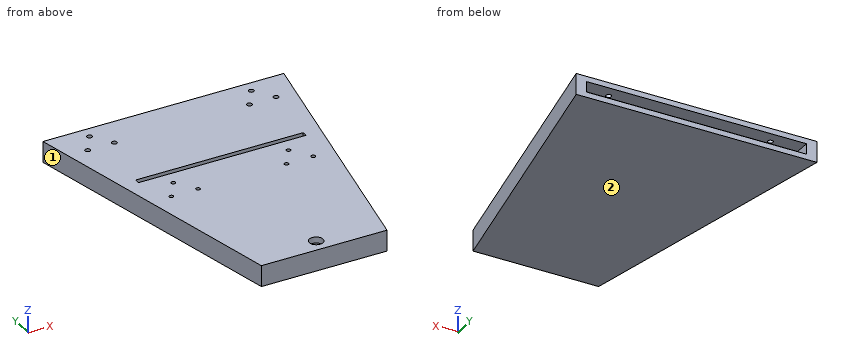
```python
from build123d import *

# Parameters (mm, degrees)
EXTRUDE_1_DEPTH     = 20
SKETCH_3_W          = 210
SKETCH_3_H          = 10
CUT_EXTRUDE_1_DEPTH = 15
SKETCH_4_W          = 160
SKETCH_4_H          = 5
CUT_EXTRUDE_2_DEPTH = 10
SKETCH_5_R          = 2.5
SKETCH_5_R_2        = 2
CUT_EXTRUDE_3_DEPTH = 10
CUT_EXTRUDE_4_DEPTH = 4.25
SKETCH_8_R          = 6.5
CUT_EXTRUDE_6_DEPTH = 15


with BuildPart() as part:
    # 草图1 → 凸台-拉伸1 (new body)
    with BuildSketch(Plane.XY):
        Polygon((-115, 220), (115, 220), (60, -50), (-60, -50), align=None)
    extrude(amount=EXTRUDE_1_DEPTH)

    # 草图3 → 切除-拉伸1 (cut)
    with BuildSketch(Plane(origin=(0, 220, 0), x_dir=(1, 0, 0), z_dir=(0, 1, 0))):
        with Locations((0, -10)):
            Rectangle(SKETCH_3_W, SKETCH_3_H)
    extrude(amount=-CUT_EXTRUDE_1_DEPTH, mode=Mode.SUBTRACT)

    # 草图4 → 切除-拉伸2 (cut)
    with BuildSketch(Plane.XY.offset(20)):
        with Locations((0, 123.51)):
            Rectangle(SKETCH_4_W, SKETCH_4_H)
    extrude(amount=-CUT_EXTRUDE_2_DEPTH, mode=Mode.SUBTRACT)

    # 草图5 → 切除-拉伸3 (cut)
    with BuildSketch(Plane.XY.offset(20)):
        with Locations((-77.25, 208.1425573)):
            Circle(SKETCH_5_R)
        with Locations((-90, 189)):
            Circle(SKETCH_5_R)
        with Locations((-64.5, 189)):
            Circle(SKETCH_5_R)
        with Locations((-55, 106.6525573)):
            Circle(SKETCH_5_R_2)
        with Locations((-67.75, 87.51)):
            Circle(SKETCH_5_R_2)
        with Locations((-42.25, 87.51)):
            Circle(SKETCH_5_R_2)
        with Locations(Location((42.25, 87.51, 0), (0, 0, 180))):
            Circle(SKETCH_5_R_2)
        with Locations(Location((67.75, 87.51, 0), (0, 0, 180))):
            Circle(SKETCH_5_R_2)
        with Locations(Location((55, 106.6525573, 0), (0, 0, 180))):
            Circle(SKETCH_5_R_2)
        with Locations(Location((64.5, 189, 0), (0, 0, 180))):
            Circle(SKETCH_5_R)
        with Locations(Location((90, 189, 0), (0, 0, 180))):
            Circle(SKETCH_5_R)
        with Locations((77.25, 208.1425573)):
            Circle(SKETCH_5_R)
    extrude(amount=-CUT_EXTRUDE_3_DEPTH, mode=Mode.SUBTRACT)

    # 草图6 → 切除-拉伸4 (cut, symmetric)
    with BuildSketch(Plane(origin=(0, 0, 10), x_dir=(-1, 0, 0), z_dir=(0, 0, -1))):
        with BuildLine():
            Line((0, -49.69), (18.016092171, -49.69))
            Line((18.016092171, -49.69), (11.781592332, -23.29))
            Line((11.781592332, -23.29), (0, -23.29))
            ThreePointArc((0, -23.29), (-13.2, -36.49), (0, -49.69))
        make_face()
    extrude(amount=CUT_EXTRUDE_4_DEPTH, both=True, mode=Mode.SUBTRACT)

    # 草图8 → 切除-拉伸6 (cut)
    with BuildSketch(Plane.XY.offset(20)):
        with Locations((0, -36.49)):
            Circle(SKETCH_8_R)
    extrude(amount=-CUT_EXTRUDE_6_DEPTH, mode=Mode.SUBTRACT)


solid = part.part
```
Build history of the part. All positions in model axes, mm. Face numbers are marked on the shaded views. Give positions to 0.01 mm unless a question says otherwise; leave off trailing zeros. Order: outer loops, then holes, each group sorted by start corner. A loop starts at its lowest first (then second) coordinate and runs counter-clockwise, first axis right, second up. Notation, with made-up numbers: M 11,65.5 L 49,65.5 A30 ccw 49,91.5 Z; hole C 13,46.5 d7. An arc over 180 degrees is marked long. Return JSON: item names as keys, results as strings.
Q1. Band-saw the part on D-D (y = 73). Give the cut face in (x, z).
Answer list:
{"outline": "M -85.06,0 L 85.06,0 L 85.06,20 L -85.06,20 Z"}
Q2. Wall check: probe 1 along Y at (x, z) = (-55, 15.5); probe 2 along X at (y, z) = (189, 17); probe 3 along Y at (x, z) = (-32.5, 9.75). Give the ranges that are in metal, low to high. Write a range as from..to.
Answer list:
{"probe 1": "y = -50..104.65, 108.65..121.01, 126.01..220", "probe 2": "x = -108.69..-92.5, -87.5..-67, -62..62, 67..87.5, 92.5..108.69", "probe 3": "y = -50..205"}
Q3. Two-plate mould, pull along X, no slides. Class the marked faces 1 and 2: pulls with the +X half, pulls with the -X half, needs draft (parallel to the pull), parting line crosses it, or undercut.
Answer list:
{"face 1": "pulls with the -X half", "face 2": "needs draft"}
Q4. Band-saw the part on A-A (x = -26). Give the cut face in (y, z).
Answer list:
{"outline": "M -50,0 L 220,0 L 220,5 L 205,5 L 205,15 L 220,15 L 220,20 L 126.01,20 L 126.01,10 L 121.01,10 L 121.01,20 L -50,20 Z"}
Q5. Flat gauge pins, fed straight in: pin 1 (1.5 mm diameter, centred on y = 122.5, z = 15, fed in from -X); pin 2 (3 mm diameter, centred on x = 36.5, z = 8.5, fed in from +Y); pin 3 (4 mm diameter, centred on y = 163.5, z = 8, fed in from +X). Where does each tip first touch, or does it go through?
Answer list:
{"pin 1": "stops at x = -95.29", "pin 2": "stops at y = 205", "pin 3": "stops at x = 103.9"}
Q6. Band-saw the part on B-B (y = -36.49). Give the cut face in (x, z).
Answer list:
{"outline": "M -62.75,0 L 62.75,0 L 62.75,20 L 6.5,20 L 6.5,14.25 L 13.2,14.25 L 13.2,5.75 L 6.5,5.75 L 6.5,5 L -6.5,5 L -6.5,5.75 L -14.9,5.75 L -14.9,14.25 L -6.5,14.25 L -6.5,20 L -62.75,20 Z"}
Q7. Band-saw the part on C-C (y = 152.5). Give the cut face in (x, z).
Answer list:
{"outline": "M -101.25,0 L 101.25,0 L 101.25,20 L -101.25,20 Z"}
